Job drawing, mm, ordinate dimensions from the low corner. One solid piece. Coordinates: 2 decimals unless noted, no trailing zeros. Write each loop counter-clockwise with the first axis right and the second up, starting at its lowest first coordinate (ties: lowest second). Pieces come first, ordered by that corner, then holes. Notation, with made-up numbers: (-14.75, -27) -> (23.25, -27) arc R25 cw to (23.25, 10) -> close; hole circle Ø4 at (23, -12). An arc over 180 degrees is marked (long way). One line per question, with ' | ' between items. Start each with the question number.
Item 1: Saw through at B-B (z = 12). List the corners of the cut face in (x, y).
Item 2: Saw through at C-C (y = 14.5). List the corners of the cut face in (x, z).
Item 3: Two-plate mould, pull along Z, no slides. Class the marked faces 1, 2, 3 and 4: pulls with the +Z half, pulls with the -Z half, needs draft (parallel to the pull), parting line crosses it, or undercut.
Item 4: Saw through at A-A (x = 15.5). List the corners of the cut face in (y, z), and give its area (3 significant figures).
Item 5: Probe probe 1 along Z at (x, y) = (15.5, 12); probe 2 along Z at (x, y) = (15.5, 9.75); probe 3 along Y at (x, z) = (27, 21.5). List the from-to ranges inside material, lowest first. Write a range as [from, to].
Item 6: Saw through at D-D (y = 4.5). List the corners of the cut face in (x, z).
Item 7: Pin check, flat tips, straight feed: pin 1 (1 mm diameter, centred on x = 0.5, y = 7, fed in from +Z); pin 2 (1.5 mm diameter, centred on y = 11.5, z = 26.5, fed in from +X); pin 3 (5 mm diameter, centred on x = 12.5, z = 10, fed in from -Y); pin 4 (2 mm diameter, centred on x = 3, z = 26.5, fed in from +Y). Stop position of each tip, or through.
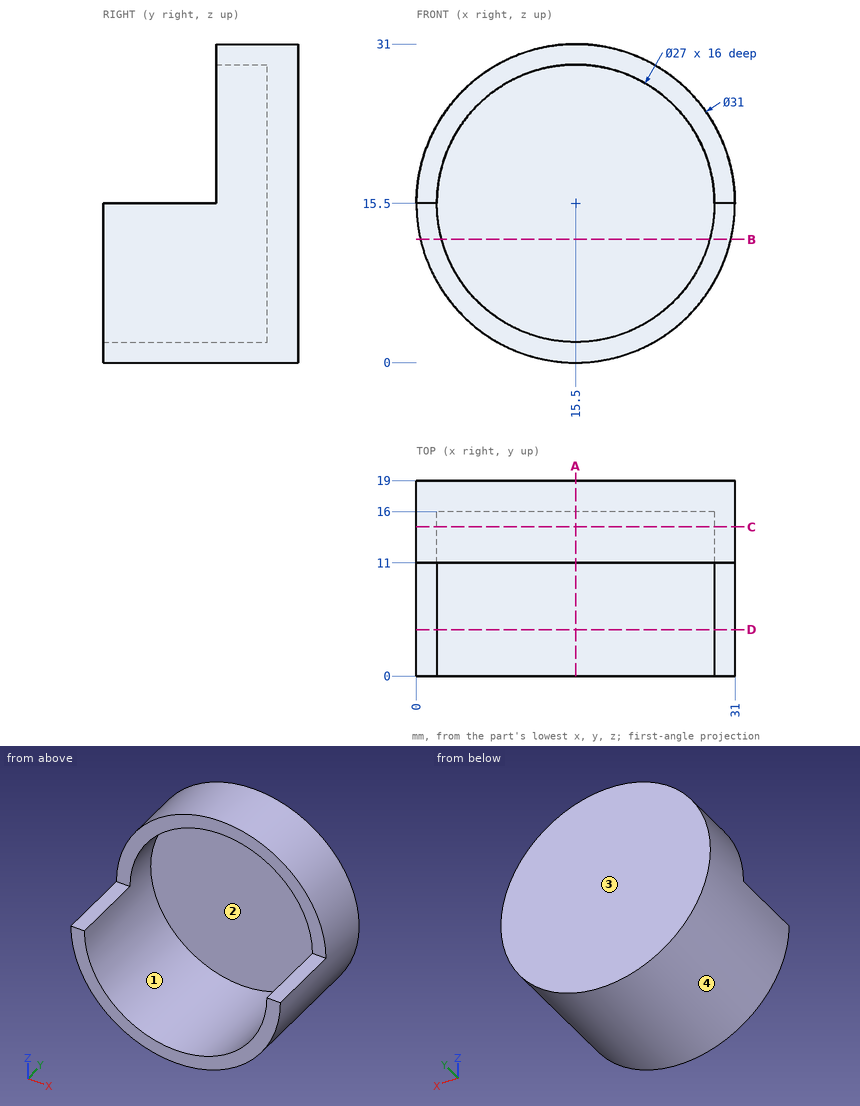
From the geometry:
1) outline: (0.4, 0) -> (2.46, 0) -> (2.46, 16) -> (28.54, 16) -> (28.54, 0) -> (30.6, 0) -> (30.6, 19) -> (0.4, 19) -> close
2) outline: circle Ø31 at (15.5, 15.5); hole circle Ø27 at (15.5, 15.5)
3) face 1: undercut | face 2: undercut | face 3: needs draft | face 4: parting line crosses it
4) outline: (0, 0) -> (19, 0) -> (19, 31) -> (11, 31) -> (11, 29) -> (16, 29) -> (16, 2) -> (0, 2) -> close | area: 135 mm2
5) probe 1: [0, 2], [29, 31] | probe 2: [0, 2] | probe 3: [16, 19]
6) outline: (0, 15.5) arc R15.5 ccw to (31, 15.5) -> (29, 15.5) arc R13.5 cw to (2, 15.5) -> close
7) pin 1: z = 15.5 | pin 2: x = 27.13 | pin 3: y = 16 | pin 4: through
